```python
from build123d import *

# Parameters (mm, degrees)
SKETCH1_W                                      = 87
SKETCH1_H                                      = 87
BOSS_EXTRUDE1_DEPTH                            = 10
BOSS_EXTRUDE1_TAPER                            = 1
CHAMFER1_SIZE                                  = 4
CHAMFER1_SIZE_2                                = 15
BOSS_EXTRUDE2_DEPTH                            = 8.5
FILLET1_R                                      = 4
CSK_FOR_M3_5_FLAT_HEAD_MACHINE_SCREW1_AT_COUNT = 2
CSK_FOR_M3_5_FLAT_HEAD_MACHINE_SCREW1_AT_PITCH = 65


with BuildPart() as part:
    # Sketch1 → Boss-Extrude1 (new body)
    with BuildSketch(Plane(origin=(0, 0, 0), x_dir=(1, 0, 0), z_dir=(0, 1, 0))):
        Rectangle(SKETCH1_W, SKETCH1_H)
    extrude(amount=BOSS_EXTRUDE1_DEPTH, taper=BOSS_EXTRUDE1_TAPER)

    # Chamfer1
    # the kernel refuses this chamfer: 15, 4 mm, written as the material it takes off along each edge
    with BuildSketch(Plane(origin=(-82.277161627, 10, 43.325449351), x_dir=(0, -0.9879836574445086, 0.1545583793347103), z_dir=(1, 0, 0)), Plane(origin=(82.277161627, 10, -43.325449351), x_dir=(0, -0.9879836574445086, -0.1545583793347103), z_dir=(-1, 0, 0))) as chamfer1_piece_1:
        Polygon((CHAMFER1_SIZE * 0.990530598403, CHAMFER1_SIZE * 0.137292147002), (-CHAMFER1_SIZE_2 * 0.154558379335, CHAMFER1_SIZE_2 * 0.987983657445), (0, 0), align=None)
    extrude(amount=164.554323254, mode=Mode.SUBTRACT)

    # Sketch2 → Boss-Extrude2 (add, symmetric)
    with BuildSketch(Plane(origin=(0, 0, 0), x_dir=(0, 0, -1), z_dir=(1, 0, 0))):
        Polygon((-14, 10), (-13.428571429, 13.958973274), (14, 10), align=None)
    extrude(amount=BOSS_EXTRUDE2_DEPTH, both=True)

    # Fillet1
    fillet1_edges = [part.edges().sort_by_distance(p)[0] for p in [
        (43.325449351, 10, 0),
        (-43.325449351, 10, 0),
        (0, 10, 28.325449351),
        (0, 10, -28.325449351),
        (-43.447629488, 3.00030461, 43.447629488),
        (-43.447629488, 3.00030461, -43.447629488),
        (-43.360354164, 8.00030461, 35.860354164),
        (-43.360354164, 8.00030461, -35.860354164),
        (43.447629488, 3.00030461, -43.447629488),
        (0, 6.000609219, -43.395258976),
        (43.447629488, 3.00030461, 43.447629488),
        (43.360354164, 8.00030461, 35.860354164),
        (43.360354164, 8.00030461, -35.860354164),
        (0, 6.000609219, 43.395258976),
    ]]
    fillet(fillet1_edges, radius=FILLET1_R)

    # Sketch3 → CSK for M3.5 Flat Head Machine Screw1 (revolve, cut)
    with BuildSketch(Plane(origin=(-32.5, 10, 0), x_dir=(0, 0, 1), z_dir=(1, 0, 0))):
        Polygon((0, 0), (0, 10), (1.95, 10), (1.95, 7.15), (4.1, 5), (4.1, 0), align=None)
    csk_for_m3_5_flat_head_machine_screw1 = revolve(axis=Axis((-32.5, 16.35, 0), (0, -1, 0)), mode=Mode.SUBTRACT)

    # CSK for M3.5 Flat Head Machine Screw1 at: CSK for M3.5 Flat Head Machine Screw1 ×2
    with Locations(*[(i * CSK_FOR_M3_5_FLAT_HEAD_MACHINE_SCREW1_AT_PITCH, 0, 0) for i in range(1, CSK_FOR_M3_5_FLAT_HEAD_MACHINE_SCREW1_AT_COUNT)]):
        add(csk_for_m3_5_flat_head_machine_screw1, mode=Mode.SUBTRACT)


solid = part.part
```
For this review, take the finished solid that the model builds, in its own axes (mm). A direction names the side the tool comes from. Give positions to 0.01 mm unless a question says otherwise; leave off trailing zeros.
Item 1: The part is to be moulded in two halves that separate along Z. For faces 1 (the face through (0.55, 8.3, -34.73)), 2 (the face through (8.5, 12, 6)), 3 (the face through (36.5, 7.5, -0.9)), say which applies: +Z half, -Z half, draft (parallel to the pull), parting line (faces both ways), or undercut.
Item 2: Take a section at A-A (z = 0). Give the number of separate pieces and of enclosed holes in the cut face, and give its area (3 significant figures).
Item 3: Insertion check: P1, Ø2.5, axis at x = 32.5, z = 0, coming from the +Y side; P2, Ø13, axis at x = -32.5, z = 0, coming from the +Y side; P3, Ø6, axis at x = 31.5, y = 5, coming from the +Z side; P4, Ø4.5, axis at y = 11.5, z = 2, coming from the +X side. Each pin has a flat end and moves straight along its axis. Give the tip position at first contact, or say it passes through.
Item 4: Machinability: for faces 4 (the face through (-34.144, 1.445, 1.048)), 5 (the face through (-8.5, 12, 6)), 6 (the face through (-35.271, 7.535, -3.022)), which of the approach directions +Z, -Z, +X, -X, +Y, -Y give a long, thin tool a straight path to every point of the face, cutting with its end or side? Answer none if there is none.
Item 5: Wall thickness on probe 1 along X at (y, z) = (2.1, 0); probe 2 along X at (y, z) = (6.2, 0); probe 3 along Z at (x, y) = (32.5, 2.15): over which ranges is each line inside the solid? List them lowest first.
Established:
1. face 1: -Z half
1. face 2: draft
1. face 3: undercut
2. separate pieces: 3
2. enclosed holes: 0
2. area: 766 mm2
3. P1: passes through
3. P2: stops at y = 10
3. P3: stops at z = 43.47
3. P4: stops at x = 41.73
4. face 4: +Y, -Y
4. face 5: +Z, -Z, -X, +Y
4. face 6: +Y
5. probe 1: x = -43.46 to -34.45, -30.55 to 30.55, 34.45 to 43.46
5. probe 2: x = -43.39 to -36.6, -28.4 to 28.4, 36.6 to 43.39
5. probe 3: z = -43.46 to -1.95, 1.95 to 43.46
